from build123d import *

# Parameters (mm, degrees)
F0_R     = 12.5
F1_DEPTH = 6
F2_R     = 8
F3_DEPTH = 10
F4_R     = 3
F5_DEPTH = 25
F6_SIZE  = 1
F7_SIZE  = 0.5


with BuildPart() as f1:
    # F0 (on Front) → F1 (new body)
    with BuildSketch(Plane.XZ):
        Circle(F0_R)
    extrude(amount=F1_DEPTH)

    # F2 (on face) → F3 (join)
    with BuildSketch(Plane.XZ.offset(6)):
        Circle(F2_R)
    extrude(amount=F3_DEPTH)

    # F4 (on face) → F5 (cut)
    with BuildSketch(Plane.XZ.offset(16)):
        Circle(F4_R)
    extrude(amount=-F5_DEPTH, mode=Mode.SUBTRACT)

    # F6
    f6_edges = [f1.edges().sort_by_distance(p)[0] for p in [
        (-12.5, -6, 0),
        (-12.5, 0, 0),
    ]]
    chamfer(f6_edges, length=F6_SIZE)

    # F7
    f7_edges = [f1.edges().sort_by_distance(p)[0] for p in [
        (-8, -16, 0),
    ]]
    chamfer(f7_edges, length=F7_SIZE)


solid = f1.part
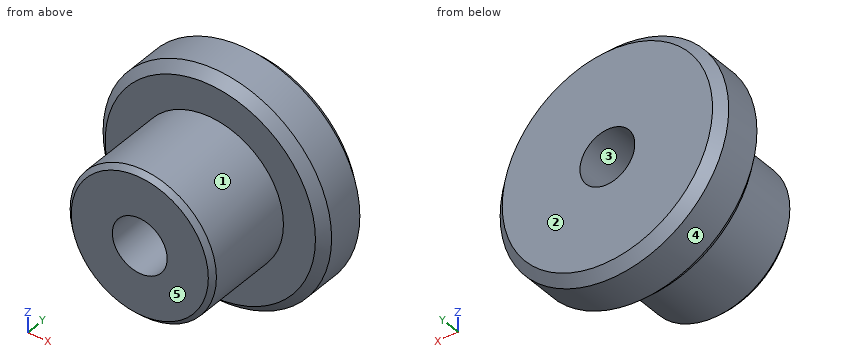
Work out the finished part from the listing and answer in its coordinate system (mm). Face numbers are marked on the shaded views. A direction names the side the tool comes from. Coordinates: 2 decimals unless noted, no trailing zeros. Loops run counter-clockwise (first coordinate to the right, second up) from the corner with the lowest first, then second, coordinate; pieces in that order, holes last. Notation, with made-up numbers: M -28.5,-5.75 L 22.5,-5.75 A37 ccw 22.5,30.25 Z; hole C 12.5,10.25 d10. An arc over 180 degrees is marked long. Answer in a Markdown table with one row per item. Add a question column.
1. Flat-ended cylindrical pins translate along their axes: P1, Ø4, axis at x = -3, z = -7, coming from the -Y side; P2, Ø1, axis at y = -2, z = -7.5, coming from the +X side; P3, Ø3, axis at x = 7, y = -10, coming from the +Z side; P4, Ø5, axis at y = -12.5, z = -7.5, coming from the +X side (3 decimals). Find the tip coordinate at first contact, or state that the pin passes through.
2. The mould has two halves that part along Z. Classify the marked faces 3, 4 and 5: pulls with the +Z half, pulls with the -Z half, needs draft (parallel to the pull), parting line crosses it, or undercut.
3. Consider L1, parallel to Z at x = 0, y = -8.75; L2, parallel to Y at x = -7.5, z = -3.25; L3, parallel to Y at x = -0.25, z = -7.5. Determine where each line is inside the solid, lowest interval first.
4. Find section A-A, the plane z = 0. Write down the section's boundary in (x, y).
5. A tool of negligible diameter and unlimited length cuts with its end or side. For the marked faces 1 and 2, from which of +Z, -Z, +X, -X, +Y, -Y can it reach the whole face along a straight path? Write none if from no direction.
6. Find section B-B, the plane x = 0. Write down the section's boundary in (y, z), then the cut area to 3 significant figures.
7. Find section C-C, the plane y = -13.5. Write down the section's boundary in (x, z).
8. Find section D-D, the plane y = -4.5. Write down the section's boundary in (x, z), then the cut area to 3 significant figures.
Reported:
| question | item | result |
|---|---|---|
| 1 | P1 | stops at y = -16 |
| 1 | P2 | stops at x = 10.36 |
| 1 | P3 | stops at z = 5.81 |
| 1 | P4 | stops at x = 6.245 |
| 2 | face 3 | undercut |
| 2 | face 4 | parting line crosses it |
| 2 | face 5 | needs draft |
| 3 | L1 | z = -8 to -3, 3 to 8 |
| 3 | L2 | y = -6 to 0 |
| 3 | L3 | y = -16 to 0 |
| 4 | outline | M -12.5,-5 L -11.5,-6 L -8,-6 L -8,-15.5 L -7.5,-16 L -3,-16 L -3,0 L -11.5,0 L -12.5,-1 Z; M 3,-16 L 7.5,-16 L 8,-15.5 L 8,-6 L 11.5,-6 L 12.5,-5 L 12.5,-1 L 11.5,0 L 3,0 Z |
| 5 | face 1 | -Y |
| 5 | face 2 | +Z, -Z, +X, -X, +Y |
| 6 | outline | M -16,-7.5 L -15.5,-8 L -6,-8 L -6,-11.5 L -5,-12.5 L -1,-12.5 L 0,-11.5 L 0,-3 L -16,-3 Z; M -16,3 L 0,3 L 0,11.5 L -1,12.5 L -5,12.5 L -6,11.5 L -6,8 L -15.5,8 L -16,7.5 Z |
| 6 | area | 212 mm^2 |
| 7 | outline | C 0,0 d16; hole C 0,0 d6 |
| 8 | outline | C 0,0 d25; hole C 0,0 d6 |
| 8 | area | 463 mm^2 |
